from build123d import *

# Parameters (mm, degrees)
SKETCH1_R               = 4.9784
BOSS_EXTRUDE1_DEPTH     = 4.826
SKETCH2_R               = 2.8829
CUT_EXTRUDE1_DEPTH      = 5.826
CUT_EXTRUDE1_DEPTH_BACK = 7.359654759
SKETCH5_R               = 6.35
CUT_EXTRUDE4_DEPTH      = 0.762
SKETCH8_W               = 25.4
SKETCH8_H               = 25.4
CUT_EXTRUDE5_DEPTH      = 9.7884001


with BuildPart() as part:
    # Sketch1 → Boss-Extrude1 (new body)
    with BuildSketch(Plane.XY):
        Circle(SKETCH1_R)
    extrude(amount=BOSS_EXTRUDE1_DEPTH)

    # Sketch3 → Revolve1 (revolve)
    with BuildSketch(Plane(origin=(0, 0, 0), x_dir=(0, 0, -1), z_dir=(1, 0, 0))):
        with BuildLine():
            Line((0, 0), (6.35, 0))
            add(Edge.make_bspline(
                [(0, 8.7884), (2.795464345, 8.743912966), (3.194527454, 4.557229334), (6.50039289, 2.137437451), (6.35, 0)],
                knots=[0, 0, 0, 0, 0.503113521, 1, 1, 1, 1], degree=3))
            Line((0, 8.7884), (0, 4.9784))
            Line((0, 4.9784), (0, 0))
        make_face()
    revolve(axis=Axis((0, 0, 0), (0, 0, -1)))

    # Sketch2 → Cut-Extrude1 (cut, two sides)
    with BuildSketch(Plane.XY) as cut_extrude1_sk:
        Circle(SKETCH2_R)
    extrude(amount=CUT_EXTRUDE1_DEPTH, mode=Mode.SUBTRACT)
    extrude(cut_extrude1_sk.sketch, amount=-CUT_EXTRUDE1_DEPTH_BACK, mode=Mode.SUBTRACT)

    # Sketch5 → Cut-Extrude4 (cut)
    with BuildSketch(Plane.XY.offset(-5.404994532)):
        Circle(SKETCH5_R)
    extrude(amount=CUT_EXTRUDE4_DEPTH, mode=Mode.SUBTRACT)

    # Sketch8 → Cut-Extrude5 (cut, through all)
    with BuildSketch(Plane(origin=(0, 0, 0), x_dir=(1, 0, 0), z_dir=(0, 1, 0))):
        Rectangle(SKETCH8_W, SKETCH8_H)
    extrude(amount=-CUT_EXTRUDE5_DEPTH, mode=Mode.SUBTRACT)


solid = part.part
Read the model definition and answer for the solid it produces. Units are mm, in the model's axes. A direction names the side the tool comes from. Coordinates: 2 decimals unless noted, no trailing zeros. Loops run counter-clockwise (first coordinate to the right, second up) from the corner with the lowest first, then second, coordinate; pieces in that order, holes last. Notation, with made-up numbers: (61, -20.75) -> (74, -20.75) arc R18 ccw to (74, -10.75) -> close; hole circle Ø1 at (83.25, 27). An arc over 180 degrees is marked (long way). Answer in a Markdown table with one row per item.
Item 1: Each of these flat-tipped pins is pushed along its axis until it touches: P1, Ø4, axis at x = -4, z = -0.5, coming from the +Y side; P2, Ø3, axis at x = 1.5, z = 3, coming from the +Y side; P3, Ø1, axis at y = 2, z = 3, coming from the +X side. Where does it stop, or does it pass through?
Returned:
| item | result |
|---|---|
| P1 | stops at y = 8.55 |
| P2 | stops at y = 4.98 |
| P3 | stops at x = 4.75 |
Item 2: Straight lines are drawn through the part: line 1 along Y through (x, z) = (-3.5, -2.25); line 2 along Y through (x, z) = (0.5, 4.25); line 3 along Z through (x, y) = (4.5, 4.75). For each, find the intervals that lie inside material, in ascending order. Write a range as [from, to].
Returned:
| item | result |
|---|---|
| line 1 | y = [0, 7.17] |
| line 2 | y = [2.84, 4.95] |
| line 3 | z = [-3.19, 0] |
Item 3: For faces 1 (the flat face through (-5, 0, -1)), 2 (the flat face through (0.1, 5.3, 0)), determine the directions among +Z, -Z, +X, -X, +Y, -Y from which every point of the face is accessible in a straight line to the end or side of a thin tool.
Returned:
| item | result |
|---|---|
| face 1 | +Z, -Z, +X, -X, -Y |
| face 2 | +Z, +Y |
Item 4: A cutting plane is placed at A-A on z = 1.25. Determine the outline of the cut face in (x, y), plus the area to 3 significant figures.
Returned:
| item | result |
|---|---|
| outline | (-4.98, 0) -> (-2.88, 0) arc R2.88 cw to (2.88, 0) -> (4.98, 0) arc R4.98 ccw to start |
| area | 25.9 mm^2 |
